Build history of the part. All positions in model axes, mm. Face numbers are marked on the shaded views. A direction names the side the tool comes from. Give positions to 0.01 mm unless a question says otherwise; leave off trailing zeros. Order: outer loops, then holes, each group sorted by start corner. A loop starts at its lowest first (then second) coordinate and runs counter-clockwise, first axis right, second up. Notation, with made-up numbers: M -34,7.5 L -12,7.5 A32 ccw -12,42.5 Z; hole C 70.25,69 d11. An arc over 180 degrees is marked long. One line per item, written item: value. Start each with the question number.
from build123d import *

# Parameters (mm, degrees)
F0_W         = 25.4
F0_H         = 25.4
F1_DEPTH     = 46.86
F3_DEPTH     = 11.11
F4_T4_ANGLE  = 22.8192997927
F4_T10_ANGLE = 22.8192997927
F4_T16_ANGLE = 22.8192997927
F4_T22_ANGLE = 22.8192997927
F5_R         = 2.2479
F6_DEPTH     = 6.4371526241
F8_R         = 9.525
F9_DEPTH     = 31.75
F10_R        = 1.4224
F11_DEPTH    = 7.9502
F7_R         = 11.303
F12_DEPTH    = 25.401
F7_R_2       = 1.4224
F13_DEPTH    = 2.5348692
F14_R        = 3.9751
F15_DEPTH    = 6.35
F16_R        = 1.4224
F17_DEPTH    = 5.715


# Not quite as in the source:
# - a fillet or chamfer that OpenCascade refuses, or shapes differently, is made with other operations: its cross-section is extruded or revolved along the edge and cut away or added


with BuildPart() as f1:
    # F0 (on Top) → F1 (new body)
    with BuildSketch(Plane.XY):
        Rectangle(F0_W, F0_H)
    extrude(amount=F1_DEPTH)

    # F2 (on face) → F3 (cut)
    with BuildSketch(Plane.XY.offset(46.86)):
        with BuildLine():
            ThreePointArc((-11.5104126772, -12.7), (-12.1198102295, -12.1198102295), (-12.7, -11.5104126772))
            Line((-12.7, -11.5104126772), (-12.7, -12.7))
            Line((-12.7, -12.7), (-11.5104126772, -12.7))
        make_face()
        with BuildLine():
            ThreePointArc((-12.7, 11.5104126772), (-12.1198102295, 12.1198102295), (-11.5104126772, 12.7))
            Line((-11.5104126772, 12.7), (-12.7, 12.7))
            Line((-12.7, 12.7), (-12.7, 11.5104126772))
        make_face()
        with BuildLine():
            Line((12.7, 12.7), (11.5104126772, 12.7))
            ThreePointArc((11.5104126772, 12.7), (12.1198102295, 12.1198102295), (12.7, 11.5104126772))
            Line((12.7, 11.5104126772), (12.7, 12.7))
        make_face()
        with BuildLine():
            Line((12.7, -12.7), (12.7, -11.5104126772))
            ThreePointArc((12.7, -11.5104126772), (12.1198102295, -12.1198102295), (11.5104126772, -12.7))
            Line((11.5104126772, -12.7), (12.7, -12.7))
        make_face()
    extrude(amount=-F3_DEPTH, mode=Mode.SUBTRACT)

    # F4: chamfer of 1 on 4 edges, made by hand


with BuildPart() as f4_tool2:
    # F4_s3 → F4_t4 (revolve)
    with BuildSketch(Plane(origin=(0, 0, 0), x_dir=(0, 0, 1), z_dir=(0.8330144325, -0.5532512587, 0))):
        Polygon((36.75, 17.14), (35.75, 18.14), (35.75, 17.14), align=None)
    revolve(axis=Axis((0, 0, 35.75), (0, 0, -1)), revolution_arc=F4_T4_ANGLE)

    split(bisect_by=Plane.XZ.offset(12.7), keep=Keep.BOTTOM)

    split(bisect_by=Plane.YZ.offset(-12.7), keep=Keep.TOP)


with BuildPart() as f1_1:
    add(f1.part)

    # F4_t1: union F4_tool2
    add(f4_tool2.part)


with BuildPart() as f4_tool8:
    # F4_s9 → F4_t10 (revolve)
    with BuildSketch(Plane(origin=(0, 0, 0), x_dir=(0, 0, 1), z_dir=(0.5532512587, 0.8330144325, 0))):
        Polygon((35.75, 18.14), (36.75, 17.14), (35.75, 17.14), align=None)
    revolve(axis=Axis((0, 0, 35.75), (0, 0, -1)), revolution_arc=F4_T10_ANGLE)

    split(bisect_by=Plane.XZ.offset(12.7), keep=Keep.BOTTOM)

    split(bisect_by=Plane.YZ.offset(12.7), keep=Keep.BOTTOM)


with BuildPart() as f1_2:
    add(f1_1.part)

    # F4_t7: union F4_tool8
    add(f4_tool8.part)


with BuildPart() as f4_tool14:
    # F4_s15 → F4_t16 (revolve)
    with BuildSketch(Plane(origin=(0, 0, 0), x_dir=(0, 0, 1), z_dir=(-0.8330144325, 0.5532512587, 0))):
        Polygon((35.75, 18.14), (36.75, 17.14), (35.75, 17.14), align=None)
    revolve(axis=Axis((0, 0, 35.75), (0, 0, -1)), revolution_arc=F4_T16_ANGLE)

    split(bisect_by=Plane.YZ.offset(12.7), keep=Keep.BOTTOM)

    split(bisect_by=Plane.XZ.offset(-12.7), keep=Keep.TOP)


with BuildPart() as f1_3:
    add(f1_2.part)

    # F4_t13: union F4_tool14
    add(f4_tool14.part)


with BuildPart() as f4_tool20:
    # F4_s21 → F4_t22 (revolve)
    with BuildSketch(Plane(origin=(0, 0, 0), x_dir=(0, 0, 1), z_dir=(-0.5532512587, -0.8330144325, 0))):
        Polygon((36.75, 17.14), (35.75, 18.14), (35.75, 17.14), align=None)
    revolve(axis=Axis((0, 0, 35.75), (0, 0, -1)), revolution_arc=F4_T22_ANGLE)

    split(bisect_by=Plane.YZ.offset(-12.7), keep=Keep.TOP)

    split(bisect_by=Plane.XZ.offset(-12.7), keep=Keep.TOP)


with BuildPart() as f1_4:
    add(f1_3.part)

    # F4_t19: union F4_tool20
    add(f4_tool20.part)

    # F5 (on face) → F6 (cut)
    with BuildSketch(Plane(origin=(-12.7, 0, 0), x_dir=(0, -1, 0), z_dir=(-1, 0, 0))):
        with Locations((0, 43.812)):
            Circle(F5_R)
    extrude(amount=-F6_DEPTH, mode=Mode.SUBTRACT)

    # F8 (on face) → F9 (cut)
    with BuildSketch(Plane.XY.offset(46.86)):
        Circle(F8_R)
    extrude(amount=-F9_DEPTH, mode=Mode.SUBTRACT)

    # F10 (on face) → F11 (cut)
    with BuildSketch(Plane.XY.offset(46.86)):
        with Locations((10.1092, -10.1092)):
            Circle(F10_R)
        with Locations((10.1092, 10.1092)):
            Circle(F10_R)
        with Locations((-10.1092, 10.1092)):
            Circle(F10_R)
        with Locations((-10.1092, -10.1092)):
            Circle(F10_R)
    extrude(amount=-F11_DEPTH, mode=Mode.SUBTRACT)

    # F7 (on face) → F12 (cut, through all)
    with BuildSketch(Plane.XZ.offset(12.7)):
        with Locations((0, 12.7)):
            Circle(F7_R)
    extrude(amount=-F12_DEPTH, mode=Mode.SUBTRACT)

    # F7 (on face) → F13 (cut)
    with BuildSketch(Plane.XZ.offset(12.7)):
        with Locations((10.1092, 22.8092)):
            Circle(F7_R_2)
        with Locations((10.1092, 2.5908)):
            Circle(F7_R_2)
        with Locations((-10.1092, 2.5908)):
            Circle(F7_R_2)
        with Locations((-10.1092, 22.8092)):
            Circle(F7_R_2)
    extrude(amount=-F13_DEPTH, mode=Mode.SUBTRACT)

    # F14 (on face) → F15 (cut)
    with BuildSketch(Plane.YZ.offset(12.7)):
        with Locations((0, 39.494)):
            Circle(F14_R)
    extrude(amount=-F15_DEPTH, mode=Mode.SUBTRACT)

    # F16 (on face) → F17 (cut)
    with BuildSketch(Plane(origin=(0, 12.7, 0), x_dir=(-1, 0, 0), z_dir=(0, 1, 0))):
        with Locations((-10.1092, 22.8092)):
            Circle(F16_R)
        with Locations((10.1092, 22.8092)):
            Circle(F16_R)
        with Locations((10.1092, 2.5908)):
            Circle(F16_R)
        with Locations((-10.1092, 2.5908)):
            Circle(F16_R)
    extrude(amount=-F17_DEPTH, mode=Mode.SUBTRACT)


solid = f1_4.part
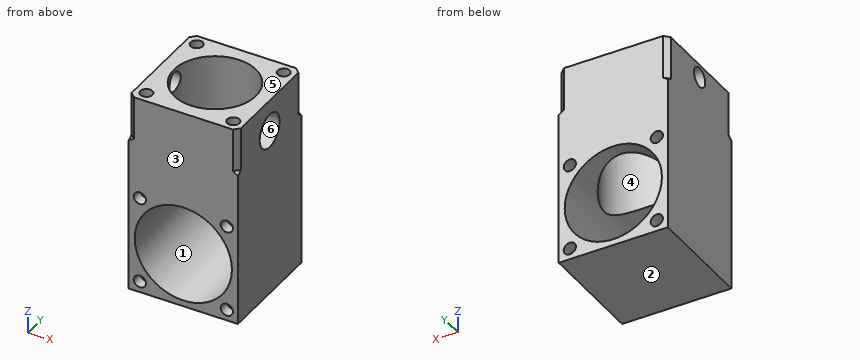
1) Slice it at D-D (z = 28). List the corners of the cut face in (x, y) (3 decimals), plus the area to 3 significant figures.
2) Pull direction Z, two halves, no side cores. Call the marked faces 1, 2 and 3: pulls with the +Z half, pulls with the -Z half, needs draft (parallel to the pull), parting line crosses it, or undercut.
3) Drill centre lines: line 1 (Y direction, x = 9, z = 41); line 2 (X direction, y = 9, z = 22); line 3 (Y direction, x = 0, z = 34.5) (3 decimals). Where is each one in solid material? Low to high.
4) Drop flat-ended pins along their axis: P1, Ø3, axis at x = -4.5, y = 4, coming from the -Z side; P2, Ø1.7, axis at x = 10.11, z = 2.59, coming from the +Y side (3 decimals); P3, Ø2.5, axis at x = 10.11, z = 22.81, coming from the -Y side; P4, Ø4, axis at y = 0, z = 43.812, coming from the -X side. Give the stop position or say it passes through.
5) Tool access for the marked faces 4, 5 and 6: list every direction of +Z, -Z, +X, -X, +Y, -Y with a clear straight run to the whole face (end or side of a thin tool).
6) Slice it at A-A (x = 0). List the corners of the cut face in (y, z) (3 decimals), plus the area to 3 significant figures.
7) Slice it at B-B (z = 12.7). List the corners of the cut face in (x, y), plus the area to 3 significant figures.
8) Slice it at C-C (y = 0). List the corners of the cut face in (x, z) (3 decimals).
Results list:
1. outline: M -12.7,-12.7 L 12.7,-12.7 L 12.7,12.7 L -12.7,12.7 Z; hole C 0,0 d19.05
1. area: 360 mm²
2. face 1: undercut
2. face 2: pulls with the -Z half
2. face 3: needs draft
3. line 1: y = -12.7 to -11, -9.22 to -3.68, 3.68 to 9.22, 11 to 12.7
3. line 2: x = -12.7 to -11.28, -8.94 to -6.42, 6.42 to 8.94, 11.28 to 12.7
3. line 3: y = -12.7 to -9.525, 9.525 to 12.7
4. P1: stops at z = 0
4. P2: stops at y = 6.985
4. P3: stops at y = -10.17
4. P4: stops at x = 9.31
5. face 4: +Z
5. face 5: +Z, +X, -X, +Y, -Y
5. face 6: +X
6. outline: M -12.7,0 L 12.7,0 L 12.7,1.397 L -12.7,1.397 Z; M -12.7,24.003 L -9.525,24.003 L -9.525,46.86 L -12.7,46.86 Z; M 9.525,24.003 L 12.7,24.003 L 12.7,46.86 L 9.525,46.86 Z
6. area: 181 mm²
7. outline: M -12.7,-12.7 L -11.3,-12.7 L -11.3,12.7 L -12.7,12.7 Z; M 11.3,-12.7 L 12.7,-12.7 L 12.7,12.7 L 11.3,12.7 Z
7. area: 71.0 mm²
8. outline: M -12.7,0 L 12.7,0 L 12.7,35.519 L 9.525,35.519 L 9.525,18.785 A11.303 cw long -9.525,18.785 L -9.525,41.564 L -12.7,41.564 Z; M -12.7,46.06 L -9.525,46.06 L -9.525,46.86 L -12.7,46.86 Z; M 9.525,43.469 L 12.7,43.469 L 12.7,46.86 L 9.525,46.86 Z
